Autodesk Inventor part; units mm, degrees
ref_plane "Plano de correa" through (0, 55, 10) normal (0, 0, 1) x (1, 0, 0)
ref_plane "YZ Plane" through (0, 0, 0) normal (1, 0, 0) x (0, 1, 0)
ref_plane "XZ Plane" through (0, 0, 0) normal (0, 1, 0) x (-1, 0, 0)
sketch "Boceto principal" plane through (0, 0, 0) normal (1, 0, 0) x (0, 1, 0)
  line L0 (0, 20) -> (68.8, 20)
  line L1 (68.8, 20) -> (68.8, 16.356)
  line L2 (68.8, 16.356) -> (55, 12.137)
  line L3 (55, 12.137) -> (55, 7.863)
  line L4 (55, 7.863) -> (68.8, 3.644)
  line L5 (68.8, 3.644) -> (68.8, 0)
  line L6 (68.8, 0) -> (0, 0)
  line L7 (66, 15.5) -> (66, 4.5) construction
  line L8 (55, 10) -> (66, 10) construction
  line L9 (68.8, 16.356) -> (68.8, 3.644)
  line L10 (0, -4) -> (0, 24)
  line L11 (0, 0) -> (0, 20)
  dimension "d0" = 11
  dimension "d1" = 34
  dimension "d2" = 2.8
  dimension "d6" = 20
  dimension "d21" = 132
  dimension "d25" = 13.8
  dimension "d27" = 10
ref_plane "Plano de correa" through (0, 55, 10) normal (0, 0, 1) x (1, 0, 0)
revolve "Cuerpo" add sketch "Boceto principal" angle 360 about axis through (0, 0, -10) along (0, 0, 1)
revolve "Para ranuras" cut sketch "Boceto principal" angle 360 about axis through (0, 0, -10) along (0, 0, 1) contours L9 L4 L3 L2
fillet "Empalme externo" [suppressed]
fillet "Empalme interno" [suppressed]
pattern_of_one "Patrón para ranuras"
sketch "Boceto2" plane through (0, 0, 20) normal (0, 0, 1) x (1, 0, 0)
  arc A0 (-14.0634, -2.5203) -> (-14.0634, 2.5203) centre (0, 0) ccw
  line L0 (-17.7165, -3.175) -> (-13.9303, -3.175)
  line L1 (-13.9303, 3.175) -> (-17.7165, 3.175)
  line L2 (-17.7165, 3.175) -> (-17.7165, -3.175)
  line L3 (-17.7165, -3.175) -> (17.7165, 3.175) construction
  line L4 (17.7165, -3.175) -> (-17.7165, 3.175) construction
  dimension "d28" = 28.575
extrude "Extrusión1" cut sketch "Boceto2" against normal blind 20
equation "\"d0\" = da_Bw"
equation "\"d1\" = da_Alfa"
equation "\"d2\" = da_c"
equation "\"d21\" = da_Dw"
equation "\"d25\" = da_Hd"
equation "\"d27\" = da_Se"
equation "\"da_r1\" = 0"
equation "\"da_r2\" = 0"
equation "\"d18\" = da_Sg"
equation "\"da_Bw\" = 11"
equation "\"da_Alfa\" = 34deg"
equation "\"da_c\" = 2.8"
equation "\"da_Dw\" = 132"
equation "\"da_Hd\" = 13.8"
equation "\"da_Se\" = 10"
equation "\"da_Sg\" = 15"
properties part number "Polea ranurada1" material "Steel"
Source: CAD feature listing. Evaluate the final solid. Frame: model axes, mm. A direction names the side the tool comes from. Coordinates: 2 decimals unless noted, no trailing zeros. Loops run counter-clockwise (first coordinate to the right, second up) from the corner with the lowest first, then second, coordinate; pieces in that order, holes last. Notation, with made-up numbers: M 59,79 L 102,79 A17 ccw 102,86 Z; hole C 75.5,31.25 d2. An arc over 180 degrees is marked long. Use a Markdown table: item, result. Add a question column.
Q1. Draft query along Y for faces 4 (the flat face through (-16, -3.175, 10)), 5 (the cylindrical face through (3.025, -68.733, 1.796)), 6 (the flat face through (-1, -16, 0)). Return one class per face: pulls with the +Y half, pulls with the -Y half, needs draft (parallel to the pull), parting line crosses it, or undercut.
Q2. Access query for faces 1 (the cylindrical face through (-53.692, -11.923, 9.97)), 2 (the flat face through (-17.716, 0, 10)), 3 (the flat face through (-1, -16, 20)). Directions: +Z, -Z, +X, -X, +Y, -Y. A direction counts if a zero-diameter tool reaches every point of the face in a straight line with its end or side. Return the directions, or none.
Q3. Material intervals for L1, parallel to Y at x = 0, z = 9.5; L2, parallel to X at y = 0, z = 9.25; L3, parallel to Z at x = -35, y = -47, sorted ascending.
Q4. Section query B-B, the plane y = 0. Return loops of the section in (x, z), and give its area (3 significant figures).
Q5. Section query C-C, the plane z = 10.25. Return loops of the section in (x, y) (1 decimal), and give its area (3 significant figures).
Q6. Section query A-A, the plane x = 0. Return loops of the section in (y, z), and give its area (3 significant figures).
Q7. First-contact query: pin 1 (8 mm diameter, centred on y = 17, z = 12.5, fed in from +X); pin 2 (12 mm diameter, centred on x = -19, z = 15.5, fed in from -Y); pin 3 (2 mm diameter, centred on x = -3.5, z = 17.5, fed in from +Y). Flat tips, straight axial feed; report the tip coordinate or a pass-through.
Result:
| question | item | result |
|---|---|---|
| 1 | face 4 | undercut |
| 1 | face 5 | parting line crosses it |
| 1 | face 6 | needs draft |
| 2 | face 1 | none |
| 2 | face 2 | +Z, -Z |
| 2 | face 3 | +Z, +X, -X, +Y, -Y |
| 3 | L1 | y = -55 to -14.29, 14.29 to 55 |
| 3 | L2 | x = -55 to -17.72, 14.29 to 55 |
| 3 | L3 | z = 0 to 6.76, 13.24 to 20 |
| 4 | outline | M -68.8,0 L -17.72,0 L -17.72,20 L -68.8,20 L -68.8,16.36 L -55,12.14 L -55,7.86 L -68.8,3.64 Z; M 14.29,0 L 68.8,0 L 68.8,3.64 L 55,7.86 L 55,12.14 L 68.8,16.36 L 68.8,20 L 14.29,20 Z |
| 4 | area | 1,880 mm2 |
| 5 | outline | C 0,0 d110; hole M -17.7,-3.2 L -13.9,-3.2 A14.3 ccw long -13.9,3.2 L -17.7,3.2 Z |
| 5 | area | 8,840 mm2 |
| 6 | outline | M -68.8,0 L -14.29,0 L -14.29,20 L -68.8,20 L -68.8,16.36 L -55,12.14 L -55,7.86 L -68.8,3.64 Z; M 14.29,0 L 68.8,0 L 68.8,3.64 L 55,7.86 L 55,12.14 L 68.8,16.36 L 68.8,20 L 14.29,20 Z |
| 6 | area | 1,950 mm2 |
| 7 | pin 1 | stops at x = 66.93 |
| 7 | pin 2 | stops at y = -67.55 |
| 7 | pin 3 | stops at y = 68.75 |
